Could you check a few things on this model? Use its own coordinates, in mm. A direction names the side the tool comes from. Coordinates: 2 decimals unless noted, no trailing zeros. Write each loop counter-clockwise with the first axis right and the second up, starting at its lowest first coordinate (ties: lowest second). Pieces come first, ordered by that corner, then holes. Notation, with made-up numbers: M -9.75,-23.5 L 16.25,-23.5 A23 ccw 16.25,9.5 Z; hole C -34,-2 d11. An arc over 180 degrees is marked long. Answer as CSV lines item,"result". Start each with the question number.
Item 1: If I drill on line 1 along Y through (x, z) = (195, 3.5); line 2 along Y through (x, z) = (91, 7); line 3 along X through (y, z) = (82, 10.25), over which ranges is the centre line in solid material (lowest first)? Write a range as [from, to].
Item 2: Suppose I cut it at B-B, the plane y = 100.5. Write out the boundary of the cut face in (x, z).
Item 3: Suppose I cut it at A-A, the plane z = 7.25. Write out the boundary of the cut face in (x, y), and give its area (3 significant figures).
Item 4: Suppose I cut it at C-C, the plane x = 160. Write out the boundary of the cut face in (y, z).
Item 5: On a 3-axis mill with a long thin cutter (end or side, diameter ignored), from which of +Z, -Z, +X, -X, +Y, -Y can I reach the whole of each face in a straight line? I mean faces 1 (the flat face through (29, 58, 12.934)), 2 (the flat face through (-140, 50, 7)), 3 (the flat face through (203, 51.07, 7)). Say none if no direction works.
Item 6: I'm going to push flat-ended pins straight in: P1, Ø1, axis at x = -35.5, z = 2, coming from the -Y side; P2, Ø6.5, axis at x = -138, z = 8, coming from the +Y side; P3, Ø1, axis at y = 81, z = 7, coming from the -X side; P4, Ø10.5, axis at x = -49.77, y = 133.39, coming from the -Z side. Where does each tip first touch, or does it pass through?
Item 7: We'd pull the mould along X, two halves only. Please class faces 4 (the flat face through (32, 147.299, 7)), 5 (the flat face through (233.044, 25, 7)), 6 (the cylindrical face through (122.239, 129.666, 6.376)), 7 (the cylindrical face through (-50.635, 129.488, 6.376)): +X half, -X half, draft (parallel to the pull), parting line (faces both ways), or undercut.
```python
from build123d import *

# Parameters (mm, degrees)
SKETCH1_R                = 3.817508494
SKETCH1_R_2              = 4
BOSS_EXTRUDE1_DEPTH      = 12.933846798
BOSS_EXTRUDE1_DEPTH_BACK = 0.0001


with BuildPart() as part:
    # Sketch1 → Boss-Extrude1 (new body, two sides)
    with BuildSketch(Plane.XY) as boss_extrude1_sk:
        Polygon((171.212226028, 51.069530268), (136.012624897, 147.29914138), (-75.017990846, 147.29914138), (-110.431982128, 50), (-169.555830253, 50), (-169.555830253, 0), (233.044157252, -0.895163773), (233.044157252, 51.069530268), align=None)
        with Locations((123.066759463, 133.392636667)):
            Circle(SKETCH1_R, mode=Mode.SUBTRACT)
        with Locations((-49.767828392, 133.392636667)):
            Circle(SKETCH1_R_2, mode=Mode.SUBTRACT)
    extrude(amount=BOSS_EXTRUDE1_DEPTH)
    extrude(boss_extrude1_sk.sketch, amount=-BOSS_EXTRUDE1_DEPTH_BACK)


solid = part.part
```
Ans:
1,line 1,"y = [-0.81, 51.07]"
1,line 2,"y = [-0.58, 147.3]"
1,line 3,"x = [-98.78, 159.9]"
2,outline,"M -92.05,0 L 153.13,0 L 153.13,12.93 L -92.05,12.93 Z"
3,outline,"M -169.56,0 L 233.04,-0.9 L 233.04,51.07 L 171.21,51.07 L 136.01,147.3 L -75.02,147.3 L -110.43,50 L -169.56,50 Z; hole C -49.77,133.39 d8; hole C 123.07,133.39 d7.64"
3,area,"44,300 mm^2"
4,outline,"M -0.73,0 L 81.72,0 L 81.72,12.93 L -0.73,12.93 Z"
5,face 1,"+Z, +X, -X, +Y, -Y"
5,face 2,"+Z, -Z, -X, +Y"
5,face 3,"+Z, -Z, +X, +Y"
6,P1,"stops at y = -0.3"
6,P2,"stops at y = 50"
6,P3,"stops at x = -99.33"
6,P4,"stops at z = 0"
7,face 4,"draft"
7,face 5,"+X half"
7,face 6,"undercut"
7,face 7,"undercut"
